Autodesk Inventor part; units mm, degrees
ref_plane "Work Plane1" through (0, 0, 5) normal (0, 0, 1) x (1, 0, 0)
ref_plane "YZ Plane" through (0, 0, 0) normal (1, 0, 0) x (0, 1, 0)
ref_plane "XZ Plane" through (0, 0, 0) normal (0, 1, 0) x (-1, 0, 0)
sketch "Sketch1" plane through (0, 0, 0) normal (0, 0, 1) x (1, 0, 0)
  line L0 (0, 0) -> (0, 12)
  line L1 (15, 0) -> (-15, 0)
  line L2 (-15, 0) -> (-15, 12)
  line L3 (-15, 12) -> (15, 12)
  line L4 (15, 12) -> (15, 0)
  line L5 (-15, 12) -> (-15, 16)
  line L6 (15, 12) -> (15, 16)
  arc A0 (-15, 16) -> (15, 16) centre (0, 53.081) ccw
  point P0 (0, 12)
  dimension "d0" = 12
  dimension "d1" = 30
  dimension "d2" = 4
  dimension "d3" = 4
  dimension "d4" = 40
extrude "Extrusion1" add sketch "Sketch1" along normal blind 10
fillet "Fillet1" radius 2 8 edges at (-15, 16, 5) (15, 16, 5) (0, 13.081, 10) (0, 13.081, 0) (15, 8, 10) (-15, 8, 10) (15, 8, 0) (-15, 8, 0)
ref_plane "Work Plane1" through (0, 0, 5) normal (0, 0, 1) x (1, 0, 0)
sketch "Sketch2" plane through (0, 0, 5) normal (0, 0, 1) x (1, 0, 0)
  line L0 (-13, 0) -> (13, 0)
  line L1 (-2.5, 0) -> (2.5, 0)
  line L2 (-1.6, 15) -> (1.6, 15)
  line L3 (-1.6, 15) -> (-2.5, 0)
  line L4 (1.6, 15) -> (2.5, 0)
  line L5 (-2.32, 3) -> (2.32, 3)
  line L6 (-2.32, 0) -> (2.32, 0)
  line L7 (-1.6, 12) -> (1.6, 12)
  line L8 (-1.6, 12) -> (-2.32, 0)
  line L9 (2.32, 0) -> (1.6, 12)
  point P0 (0, 0)
  point P1 (0, 0)
  point P2 (0, 15)
  point P3 (0, 0)
  point P4 (0, 12)
  dimension "d9" = 5
  dimension "d10" = 2.5
  dimension "d11" = 3.2
  dimension "d13" = 12
  dimension "d14" = 4.64
  dimension "d15" = 4.64
  dimension "d16" = 2.32
  dimension "d17" = 3.2
  dimension "d18" = 12
extrude "Extrusion2" cut sketch "Sketch2" along normal mid plane 0.6 contours L8 L5 L9 L0 | L8 L7 L9 L5
properties part number "pot slider" material "ABS Plastic"
Read the model definition and answer for the solid it produces. Units are mm, in the model's axes. A direction names the side the tool comes from. Round coordinates to 2 decimals unless told otherwise and drop trailing zeros. Loops run counter-clockwise (first coordinate to the right, second up) from the corner with the lowest first, then second, coordinate; pieces in that order, holes last.
Q1. Determine the mould class of faces 1 (the face through (0, 7, 0)), 2 (the face through (14.4, 6.66, 9.43)), 3 (the face through (0.18, 13.08, 4.96)) for opening direction X: released by +X, released by -X, zero draft, split by the parting line, or undercut.
Q2. Consider probe 1 along Z at (x, y) = (-1.25, 2.25); probe 2 along Y at (x, z) = (-13, 1.25); probe 3 along Y at (x, z) = (2.5, 7). Determine where each line is inside the solid, lowest interval first.
Q3. Section A-A on y = 6 is taken. Write down the section's boundary in (x, z).
Q4. Which of the six approach directions +Z, -Z, +X, -X, +Y, -Y give full straight-line access (tool end or side, diameter ignored) to faces 4 (the face through (0, 6, 5.3)), 5 (the face through (-14.43, 6.48, 0.6))?
Q5. Section C-C on y = 4.25 is taken. Write down the section's boundary in (x, z) (3 decimals).
Q6. Section B-B on z = 2.5 is taken. Write down the section's boundary in (x, y).
Q7. Section D-D on z = 9.25 is taken. Write down the section's boundary in (x, y), and give its area (3 significant figures).
Q8. Each of these flat-tipped pins is pushed along its axis until it touches: pin 1 (2 mm diameter, centred on x = 11, z = 9, fed in from +Y); pin 2 (6 mm diameter, centred on x = -9.5, z = 4, fed in from +Y). Where does it stop, or does it pass through?
Output:
1. face 1: zero draft
1. face 2: released by +X
1. face 3: undercut
2. probe 1: z = 0 to 4.7, 5.3 to 10
2. probe 2: y = 0 to 15
2. probe 3: y = 0 to 13.16
3. outline: (-15, 2) arc R2 ccw to (-13, 0) - (13, 0) arc R2 ccw to (15, 2) - (15, 8) arc R2 ccw to (13, 10) - (-13, 10) arc R2 ccw to (-15, 8) - close; hole (-1.96, 4.7) - (1.96, 4.7) - (1.96, 5.3) - (-1.96, 5.3) - close
4. face 4: -Y
4. face 5: -Z, -X, +Y, -Y
5. outline: (-15, 2) arc R2 ccw to (-13, 0) - (13, 0) arc R2 ccw to (15, 2) - (15, 8) arc R2 ccw to (13, 10) - (-13, 10) arc R2 ccw to (-15, 8) - close; hole (-2.065, 4.7) - (2.065, 4.7) - (2.065, 5.3) - (-2.065, 5.3) - close
6. outline: (-15, 0) - (15, 0) - (15, 13.14) arc R2 ccw to (12.38, 15.05) arc R40 cw to (-12.38, 15.05) arc R2 ccw to (-15, 13.14) - close
7. outline: (-14.56, 0) - (14.56, 0) - (14.56, 13.14) arc R1.56 ccw to (12.52, 14.63) arc R40.44 cw to (-12.52, 14.63) arc R1.56 ccw to (-14.56, 13.14) - close
7. area: 392 mm2
8. pin 1: stops at y = 14.82
8. pin 2: stops at y = 15.08
